CAD build for the part. Positions are in the model's coordinates, mm. Face numbers are marked on the shaded views. A direction names the side the tool comes from. Round coordinates to 2 decimals unless told otherwise and drop trailing zeros. Loops run counter-clockwise (first coordinate to the right, second up) from the corner with the lowest first, then second, coordinate; pieces in that order, holes last. Notation, with made-up numbers: M -9,14.25 L 11,14.25 A8 cw 11,18.25 Z; hole C 31,-27.75 d3. An arc over 180 degrees is marked long. One line per item, written item: value. Start each with the question number.
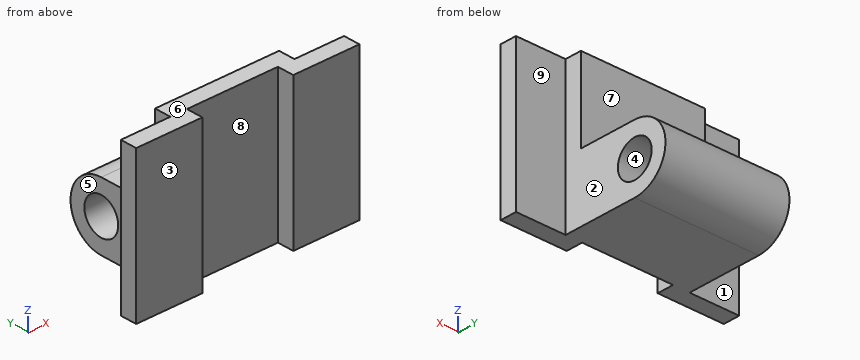
from build123d import *

# Parameters (mm, degrees)
F0_W     = 135
F0_H     = 10
F1_DEPTH = 90
F2_W     = 75
F2_H     = 90
F3_DEPTH = 10
F4_W     = 55
F4_H     = 10
F5_DEPTH = 90.001
F7_DEPTH = 75
F10_D    = 22


with BuildPart() as f1:
    # F0 (on Top) → F1 (new body)
    with BuildSketch(Plane.XY):
        with Locations((67.5, -5)):
            Rectangle(F0_W, F0_H)
    extrude(amount=F1_DEPTH)

    # F2 (on Front) → F3 (join)
    with BuildSketch(Plane.XZ):
        with Locations((67.5, 45)):
            Rectangle(F2_W, F2_H)
    extrude(amount=-F3_DEPTH)

    # F4 (on face) → F5 (cut, through all)
    with BuildSketch(Plane.XY.offset(90)):
        with Locations((67.5, -5)):
            Rectangle(F4_W, F4_H)
    extrude(amount=-F5_DEPTH, mode=Mode.SUBTRACT)

    # F6 (on face) → F7 (join)
    with BuildSketch(Plane.YZ.offset(105)):
        with BuildLine():
            Line((10, 40), (10, 0))
            Line((10, 0), (45, 0))
            ThreePointArc((45, 0), (65, 20), (45, 40))
            Line((45, 40), (10, 40))
        make_face()
    extrude(amount=-F7_DEPTH)

    # F10 (through all)
    with Locations(Plane.YZ.offset(105)):
        with Locations((45, 20)):
            Hole(F10_D / 2)


solid = f1.part
(1) Probe L1, parallel to Z at x = 76, y = 45; L2, parallel to X at y = -5.5, z = 48; L3, parallel to Y at x = 15, z = 53. List the from-to ranges inside material, lowest first.
(2) Slice it at D-D, the plane z = 78.5. List the corners of the cut face in (x, y).
(3) Mould opens along Y. For the marked faces 1, 2, 3 and 4 say: pulls with the +Y half, pulls with the -Y half, needs draft (parallel to the pull), parting line crosses it, or undercut.
(4) Slice it at C-C, the plane x = 51. List the corners of the cut face in (y, z).
(5) Slice it at A-A, the plane z = 20. List the corners of the cut face in (x, y), and give its area (4 significant figures).
(6) Which spindle directions (+Z, -Z, +X, -X, +Y, -Y) get a long thin tool onto all of the face, cutting with end or side? Do the marked faces 5, 6, 7, 8 and 9. Say none if no direction does.
(7) Flat gauge pins, fed straight in: P1, Ø16.5, axis at x = 63.5, z = 41, coming from the -Y side; P2, Ø6, axis at y = 37, z = 27, coming from the -X side; P3, Ø12, axis at y = 23, z = 18.5, coming from the +X side; P4, Ø4, axis at y = -2, z = 25.5, coming from the -X side. Where does each tip first touch, or does it go through?
(8) Slice it at B-B, the plane y = -4. List the corners of the cut face in (x, z), and give its area (3 significant figures).
Check result:
1. L1: z = 0 to 9, 31 to 40
1. L2: x = 0 to 40, 95 to 135
1. L3: y = -10 to 0
2. outline: M 0,-10 L 40,-10 L 40,0 L 95,0 L 95,-10 L 135,-10 L 135,0 L 105,0 L 105,10 L 30,10 L 30,0 L 0,0 Z
3. face 1: pulls with the +Y half
3. face 2: needs draft
3. face 3: pulls with the -Y half
3. face 4: undercut
4. outline: M 0,0 L 45,0 A20 ccw 45,40 L 10,40 L 10,90 L 0,90 Z; hole C 45,20 d22
5. outline: M 0,-10 L 40,-10 L 40,0 L 95,0 L 95,-10 L 135,-10 L 135,0 L 105,0 L 105,34 L 30,34 L 30,0 L 0,0 Z; M 30,56 L 105,56 L 105,65 L 30,65 Z
5. area: 4,025 mm^2
6. face 5: +Z, -Z, -X, +Y
6. face 6: +Z, +X, -X, +Y, -Y
6. face 7: +Z, +X, -X, +Y
6. face 8: +Z, -Z, -Y
6. face 9: +Z, -Z, +X, +Y
7. P1: stops at y = 0
7. P2: stops at x = 30
7. P3: stops at x = 105
7. P4: stops at x = 0
8. outline: M 0,0 L 40,0 L 40,90 L 0,90 Z; M 95,0 L 135,0 L 135,90 L 95,90 Z
8. area: 7,200 mm^2
